Verification items for the finished model (mm, model axes). Face numbers are marked on the shaded views. Round coordinates to 2 decimals unless told otherwise and drop trailing zeros. Order: outer loops, then holes, each group sorted by start corner. A loop starts at its lowest first (then second) coordinate and runs counter-clockwise, first axis right, second up. Notation, with made-up numbers: M 3,66 L 46,66 A9 ccw 46,78 Z; hole C -7.5,69 d8. An arc over 180 degrees is marked long. Use one line per item in the form item = value. Start each with the question number.
Item 1: Release check for a two-part mould opening along X. For the marked faces 1, 2 and 3 record: +X half, -X half, draft (parallel to the pull), parting line (faces both ways), or undercut.
Item 2: Cross-section at A-A on z = 14. Enter the section's corners in (x, y).
Item 3: Go/stop test with flat-tipped pins: pin 1 Ø1.8 at (x, z) = (-9, -5.5) entering from +Y; pin 2 Ø0.5 at (y, z) = (2, 16) entering from -X; pin 3 Ø2.5 at (x, y) = (-3.5, -1.5) entering from +Z; pin 4 Ø0.8 at (x, z) = (0, 13.5) entering from -Y. Record where each tip stops, or that it passes through.
Item 4: Cross-section at D-D on x = 3.25. Enter the section's corners in (y, z).
Item 5: Cross-section at C-C on y = 1.75. Count the separate pieces of the cut face and the enclosed holes in it, then the cut area to 3 significant figures.
Item 6: Thickness scan on probe 1 along Z at (x, y) = (-2.25, -2.5); probe 2 along Z at (x, y) = (0, -0.2); probe 3 along X at (y, z) = (0.45, -6.9). Record the ranges inside material, lowest first. Write a range as [from, to].
from build123d import *

# Parameters (mm, degrees)
SKETCH_1_W                  = 20.3
SKETCH_1_H                  = 26.6
EXTRUDE_1_DEPTH             = 5.1
HOLE_WIZARD_3_2_3_2_1_D     = 3.2
HOLE_WIZARD_2_3_2_3_1_D     = 2.3
HOLE_WIZARD_2_3_2_3_1_DEPTH = 2.3
HOLE_WIZARD_4_6_4_6_1_D     = 4.6
HOLE_WIZARD_4_6_4_6_1_DEPTH = 2.3
CHAMFER_1_SIZE              = 1
SKETCH_20_R                 = 1.6
CUT_EXTRUDE_7_DEPTH         = 1.5
SKETCH_2_W                  = 2.65
SKETCH_2_H                  = 0.7
SKETCH_2_W_2                = 3.04
EXTRUDE_2_DEPTH             = 1.5
SWEEP_START                 = -6.75
SWEEP_1_DEPTH               = 2.65
SWEEP_START_2               = -1.52
SWEEP_2_DEPTH               = 3.04
SWEEP_START_3               = 4.1
SWEEP_3_DEPTH               = 2.65
CUT_EXTRUDE_8_DEPTH         = 1
CUT_EXTRUDE_8_DEPTH_BACK    = 15.5
SKETCH_25_W                 = 1.3965698
SKETCH_25_H                 = 0.598451561
SKETCH_25_W_2               = 1.400753048
SKETCH_25_W_3               = 1.404395486
EXTRUDE_3_DEPTH             = 2.5


# Read off the part's stored shape, not the designer's step: По траектории1, По траектории2, По траектории3
with BuildPart() as part:
    # Эскиз1 → Бобышка-Вытянуть1 (new body)
    with BuildSketch(Plane(origin=(0, 2.3, 0), x_dir=(1, 0, 0), z_dir=(0, 1, 0))):
        Rectangle(SKETCH_1_W, SKETCH_1_H)
    extrude(amount=-EXTRUDE_1_DEPTH)

    # Диаметр отверстия Ø3.2 (3.2)1 (through all)
    with Locations(Plane(origin=(0, 2.3, 0), x_dir=(1, 0, 0), z_dir=(0, 1, 0))):
        with Locations((0, 6.9)):
            Hole(HOLE_WIZARD_3_2_3_2_1_D / 2)

    # Диаметр отверстия Ø2.3 (2.3)1
    with Locations(Plane(origin=(0, 2.3, 0), x_dir=(1, 0, 0), z_dir=(0, 1, 0))):
        with Locations((10.15, -1.9), (-10.15, -1.9)):
            Hole(HOLE_WIZARD_2_3_2_3_1_D / 2, depth=HOLE_WIZARD_2_3_2_3_1_DEPTH)

    # Диаметр отверстия Ø4.6 (4.6)1
    with Locations(Plane(origin=(0, 2.3, 0), x_dir=(1, 0, 0), z_dir=(0, 1, 0))):
        with Locations((10.15, 6.8), (-10.15, 6.8)):
            Hole(HOLE_WIZARD_4_6_4_6_1_D / 2, depth=HOLE_WIZARD_4_6_4_6_1_DEPTH)

    # Фаска1
    chamfer_1_edges = [part.edges().sort_by_distance(p)[0] for p in [
        (-10.15, -0.25, -13.3),
        (10.15, -0.25, -13.3),
        (10.15, -0.25, 13.3),
        (-10.15, -0.25, 13.3),
    ]]
    chamfer(chamfer_1_edges, length=CHAMFER_1_SIZE)

    # Эскиз20 → Вырез-Вытянуть7 (cut)
    with BuildSketch(Plane.XZ.offset(2.8)):
        Polygon((-8.735786438, -12.3), (8.735786438, -12.3), (9.15, -11.885786438), (9.15, 11.885786438), (8.735786438, 12.3), (-8.735786438, 12.3), (-9.15, 11.885786438), (-9.15, -11.885786438), align=None)
        with Locations(Location((0, -6.9, 0), (0, 0, 90))):
            Circle(SKETCH_20_R, mode=Mode.SUBTRACT)
    extrude(amount=-CUT_EXTRUDE_7_DEPTH, mode=Mode.SUBTRACT)

    # Эскиз2 → Бобышка-Вытянуть2 (add)
    with BuildSketch(Plane.XY.offset(13.3)):
        with Locations((-5.425, 0.35)):
            Rectangle(SKETCH_2_W, SKETCH_2_H)
        with Locations((0, 0.35)):
            Rectangle(SKETCH_2_W_2, SKETCH_2_H)
        with Locations((5.425, 0.35)):
            Rectangle(SKETCH_2_W, SKETCH_2_H)
    extrude(amount=EXTRUDE_2_DEPTH)

    # По траектории1 outline → По траектории1 (add)
    with BuildSketch(Plane.YZ.offset(SWEEP_START)):
        with BuildLine():
            Line((0.761891294, 14.869390662), (1.385375103, 15.225085604))
            Line((1.385375103, 15.225085604), (0.81420695, 15.629766886))
            Line((0.81420695, 15.629766886), (0.494271743, 15.44724517))
            Line((0.494271743, 15.44724517), (0.36086417, 15.351999112))
            ThreePointArc((0.36086417, 15.351999112), (0.144711062, 15.099351835), (0, 14.8))
            Line((0, 14.8), (0.7, 14.8))
            ThreePointArc((0.7, 14.8), (0.729738232, 14.835772255), (0.761891294, 14.869390662))
        make_face()
    extrude(amount=SWEEP_1_DEPTH)

    # По траектории2 outline → По траектории2 (add)
    with BuildSketch(Plane.YZ.offset(SWEEP_START_2)):
        with BuildLine():
            Line((0.761891294, 14.869390662), (1.385375103, 15.225085604))
            Line((1.385375103, 15.225085604), (0.81420695, 15.629766886))
            Line((0.81420695, 15.629766886), (0.494271743, 15.44724517))
            Line((0.494271743, 15.44724517), (0.36086417, 15.351999112))
            ThreePointArc((0.36086417, 15.351999112), (0.144711062, 15.099351835), (0, 14.8))
            Line((0, 14.8), (0.7, 14.8))
            ThreePointArc((0.7, 14.8), (0.729738232, 14.835772255), (0.761891294, 14.869390662))
        make_face()
    extrude(amount=SWEEP_2_DEPTH)

    # По траектории3 outline → По траектории3 (add)
    with BuildSketch(Plane.YZ.offset(SWEEP_START_3)):
        with BuildLine():
            Line((0.761891294, 14.869390662), (1.385375103, 15.225085604))
            Line((1.385375103, 15.225085604), (0.81420695, 15.629766886))
            Line((0.81420695, 15.629766886), (0.494271743, 15.44724517))
            Line((0.494271743, 15.44724517), (0.36086417, 15.351999112))
            ThreePointArc((0.36086417, 15.351999112), (0.144711062, 15.099351835), (0, 14.8))
            Line((0, 14.8), (0.7, 14.8))
            ThreePointArc((0.7, 14.8), (0.729738232, 14.835772255), (0.761891294, 14.869390662))
        make_face()
    extrude(amount=SWEEP_3_DEPTH)

    # Эскиз24 → Вырез-Вытянуть8 (cut, two sides: drawn at the far end of the back side and taken through both)
    with BuildSketch(Plane.ZY.offset(6.75).offset(-CUT_EXTRUDE_8_DEPTH_BACK)):
        Polygon((15.629766886, 0.81420695), (15.0115294, 1.166908885), (15.187532371, 1.475417638), (15.841474348, 1.102346438), (15.665471376, 0.793837685), align=None)
    extrude(amount=CUT_EXTRUDE_8_DEPTH + CUT_EXTRUDE_8_DEPTH_BACK, mode=Mode.SUBTRACT)

    # Эскиз25 → Бобышка-Вытянуть3 (add)
    with BuildSketch(Plane(origin=(0, 7.341514488, 4.188303737), x_dir=(1, 0, 0), z_dir=(0, 0.8685919072443863, 0.49552810078698817))):
        with Locations((-5.425, -12.855160228)):
            Rectangle(SKETCH_25_W, SKETCH_25_H)
        with Locations((0, -12.855160228)):
            Rectangle(SKETCH_25_W_2, SKETCH_25_H)
        with Locations((5.425, -12.855160228)):
            Rectangle(SKETCH_25_W_3, SKETCH_25_H)
    extrude(amount=EXTRUDE_3_DEPTH)


solid = part.part
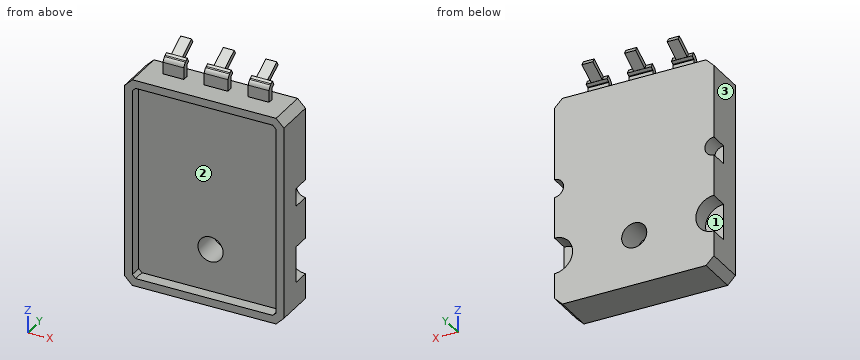
Output values:
q1.face_1 = draft
q1.face_2 = undercut
q1.face_3 = -X half
q2.outline = M -6.75,0 L -4.1,0 L -4.1,0.7 L -6.75,0.7 Z; M -1.52,0 L 1.52,0 L 1.52,0.7 L -1.52,0.7 Z; M 4.1,0 L 6.75,0 L 6.75,0.7 L 4.1,0.7 Z
q3.pin_1 = 2.3
q3.pin_2 = -6.12
q3.pin_3 = 13.3
q3.pin_4 = -2.8
q4.outline = M -2.8,-13.3 L 2.3,-13.3 L 2.3,13.3 L -2.8,13.3 L -2.8,12.3 L -1.3,12.3 L -1.3,-12.3 L -2.8,-12.3 Z
q5.separate_pieces = 4
q5.enclosed_holes = 1
q5.area = 512 mm2
q6.probe_1 = [-13.3, -12.3], [12.3, 13.3]
q6.probe_2 = [-13.3, -8.5], [-5.3, 13.3]
q6.probe_3 = [-7.85, -1.6], [1.6, 7.85]
